Part model, mm, in its own coordinate system. Face numbers are marked on the shaded views. A direction names the side the tool comes from. Give positions to 0.01 mm unless a question says otherwise; leave off trailing zeros. Order: outer loops, then holes, each group sorted by start corner. A loop starts at its lowest first (then second) coordinate and runs counter-clockwise, first axis right, second up.
from build123d import *

# Parameters (mm, degrees)
SKETCH1_W           = 74.93
SKETCH1_H           = 6.35
BOSS_EXTRUDE1_DEPTH = 3.175
SKETCH2_R           = 3.048
BOSS_EXTRUDE2_DEPTH = 5.334
SKETCH3_W           = 6.096
SKETCH3_H           = 6.096
BOSS_EXTRUDE3_DEPTH = 3.175
SKETCH4_R           = 3.048
BOSS_EXTRUDE4_DEPTH = 10.16
SKETCH5_W           = 6.096
SKETCH5_H           = 6.096
BOSS_EXTRUDE5_DEPTH = 3.175
FILLET1_R           = 0.635
FILLET2_R           = 3.175


with BuildPart() as part:
    # Sketch1 → Boss-Extrude1 (new body)
    with BuildSketch(Plane(origin=(0, 0, 0), x_dir=(1, 0, 0), z_dir=(0, 1, 0))):
        Rectangle(SKETCH1_W, SKETCH1_H)
    extrude(amount=BOSS_EXTRUDE1_DEPTH)

    # Sketch2 → Boss-Extrude2 (add)
    with BuildSketch(Plane(origin=(0, 3.175, 0), x_dir=(1, 0, 0), z_dir=(0, 1, 0))):
        with Locations(Location((-34.29, 0, 0), (0, 0, 270))):
            Circle(SKETCH2_R)
    extrude(amount=BOSS_EXTRUDE2_DEPTH)

    # Sketch3 → Boss-Extrude3 (add)
    with BuildSketch(Plane(origin=(0, 8.509, 0), x_dir=(1, 0, 0), z_dir=(0, 1, 0))):
        with Locations((-34.29, 0)):
            Rectangle(SKETCH3_W, SKETCH3_H)
    extrude(amount=BOSS_EXTRUDE3_DEPTH)

    # Sketch4 → Boss-Extrude4 (add)
    with BuildSketch(Plane(origin=(0, 3.175, 0), x_dir=(1, 0, 0), z_dir=(0, 1, 0))):
        with Locations(Location((34.29, 0, 0), (0, 0, 270))):
            Circle(SKETCH4_R)
    extrude(amount=BOSS_EXTRUDE4_DEPTH)

    # Sketch5 → Boss-Extrude5 (add)
    with BuildSketch(Plane(origin=(0, 13.335, 0), x_dir=(1, 0, 0), z_dir=(0, 1, 0))):
        with Locations((34.29, 0)):
            Rectangle(SKETCH5_W, SKETCH5_H)
    extrude(amount=BOSS_EXTRUDE5_DEPTH)

    # Fillet1
    fillet1_edges = [part.edges().sort_by_distance(p)[0] for p in [
        (-37.338, 10.0965, -3.048),
        (-37.338, 10.0965, 3.048),
        (-31.242, 10.0965, 3.048),
        (-31.242, 10.0965, -3.048),
        (37.338, 14.9225, 3.048),
        (37.338, 14.9225, -3.048),
        (31.242, 14.9225, -3.048),
        (31.242, 14.9225, 3.048),
    ]]
    fillet(fillet1_edges, radius=FILLET1_R)

    # Fillet2
    fillet2_edges = [part.edges().sort_by_distance(p)[0] for p in [
        (-37.465, 1.5875, 3.175),
        (-37.465, 1.5875, -3.175),
        (37.465, 1.5875, -3.175),
        (37.465, 1.5875, 3.175),
    ]]
    fillet(fillet2_edges, radius=FILLET2_R - 0.0001)  # a hair under: the kernel refuses the full size


solid = part.part
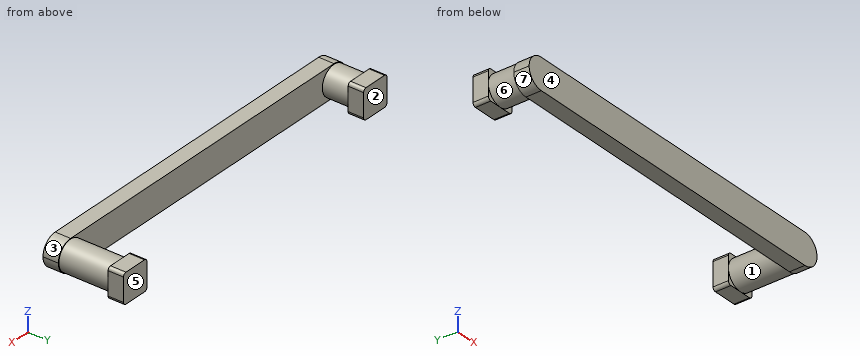
Item 1: Which spindle directions (+Z, -Z, +X, -X, +Y, -Y) get a long thin tool onto all of the face, cutting with end or side? Do the marked faces 1, 2, 3 and 4. Say none if no direction does.
Item 2: Band-saw the part on C-C on x = 14.5. List the corners of the cut face in (y, z) (3 decimals), plus the area to 3 significant figures.
Item 3: Band-saw the part on B-B on z = -1.5. List the corners of the cut face in (x, y) (3 decimals), plus the area to 3 significant figures.
Item 4: Pull direction X, two halves, no side cores. Call the marked faces 5, 6 and 7: released by +X, released by -X, zero draft, split by the parting line, or undercut.
Item 5: Drill centre lines: probe 1 along X at (y, z) = (6.5, -0.25); probe 2 along Y at (x, z) = (16, -2.25) (3 decimals); probe 3 along X at (y, z) = (9.25, 1.75). Where is each one in solid material? Low to high.
Item 6: Drop flat-ended pins along their axis: P1, Ø1.6, axis at y = 9.5, z = -1, coming from the -X side; P2, Ø2.5, axis at x = 36, z = -2, coming from the -Y side; P3, Ø1.5, axis at x = -10, z = -1, coming from the +Y side (3 decimals); P4, Ø1, axis at y = 14.5, z = 1, coming from the -X side. Give the stop position or say it passes through.
Working result:
1. face 1: none
1. face 2: +Z, -Z, -X, +Y
1. face 3: +Z, +X, -Y
1. face 4: +Z, -Z, +X, -X, -Y
2. outline: (0, -3.175) - (3.175, -3.175) - (3.175, 3.175) - (0, 3.175) - close
2. area: 20.2 mm2
3. outline: (-37.338, 8.509) - (-36.943, 8.509) - (-36.943, 3.175) - (-37.088, 3.175) - (-37.088, 0) - (37.088, 0) - (37.088, 3.175) - (36.943, 3.175) - (36.943, 13.335) - (37.338, 13.335) - (37.338, 16.51) - (31.242, 16.51) - (31.242, 13.335) - (31.637, 13.335) - (31.637, 3.175) - (-31.637, 3.175) - (-31.637, 8.509) - (-31.242, 8.509) - (-31.242, 11.684) - (-37.338, 11.684) - close
3. area: 356 mm2
4. face 5: zero draft
4. face 6: undercut
4. face 7: released by -X
5. probe 1: x = -37.33 to -31.25, 31.25 to 37.33
5. probe 2: y = 0 to 3.175
5. probe 3: x = -37.34 to -31.24, 31.79 to 36.79
6. P1: stops at x = -37.34
6. P2: stops at y = 0
6. P3: stops at y = 3.175
6. P4: stops at x = 31.24
